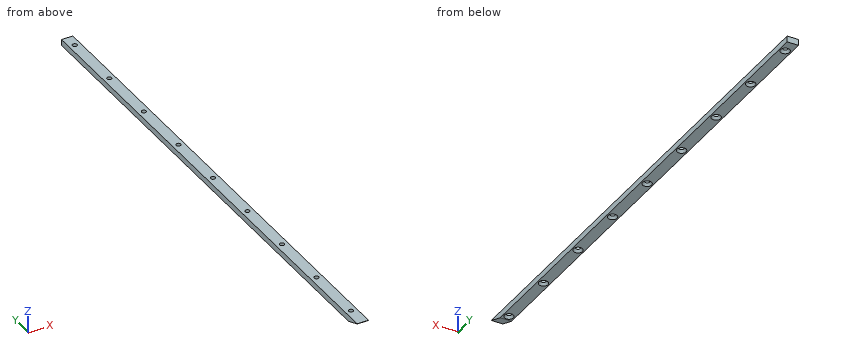
```python
from build123d import *

# Parameters (mm, degrees)
SKETCH1_W           = 15
SKETCH1_H           = 685
BOSS_EXTRUDE1_DEPTH = 4
SKETCH2_R           = 3
CUT_EXTRUDE1_DEPTH  = 8
CHAMFER1_SIZE       = 20
CHAMFER1_SIZE2      = 7.677280701
LPATTERN1_COUNT     = 9
LPATTERN1_PITCH     = 80
CHAMFER2_SIZE       = 3


with BuildPart() as part:
    # Sketch1 → Boss-Extrude1 (new, symmetric)
    with BuildSketch(Plane.XY):
        Rectangle(SKETCH1_W, SKETCH1_H)
    extrude(amount=BOSS_EXTRUDE1_DEPTH, both=True)

    # Sketch2 → Cut-Extrude1 (cut)
    with BuildSketch(Plane.XY.offset(4)):
        with Locations((0, 324.86225561)):
            Circle(SKETCH2_R)
    cut_extrude1 = extrude(amount=-CUT_EXTRUDE1_DEPTH, mode=Mode.SUBTRACT)

    # Chamfer1
    chamfer1_edges = [part.edges().sort_by_distance(p)[0] for p in [
        (0, -342.5, -4),
    ]]
    chamfer1_side = [part.faces().sort_by_distance(p)[0] for p in [
        (0, -0.896409661, -4),
    ]]
    chamfer(chamfer1_edges, length=CHAMFER1_SIZE, length2=CHAMFER1_SIZE2, reference=chamfer1_side[0])

    # LPattern1: Cut-Extrude1 ×9
    with Locations(*[(0, -i * LPATTERN1_PITCH, 0) for i in range(1, LPATTERN1_COUNT)]):
        add(cut_extrude1, mode=Mode.SUBTRACT)

    # Chamfer2
    chamfer2_edges = [part.edges().sort_by_distance(p)[0] for p in [
        (-3, 324.86225561, -4),
        (-3, 244.86225561, -4),
        (-3, 164.86225561, -4),
        (-3, 84.86225561, -4),
        (-3, 4.86225561, -4),
        (-3, -75.13774439, -4),
        (-3, -155.13774439, -4),
        (-3, -235.13774439, -4),
        (-3, -315.13774439, -4),
    ]]
    chamfer(chamfer2_edges, length=CHAMFER2_SIZE)


solid = part.part
```
Here's how the part is built. I have some questions about the finished solid (model axes, mm). Coordinates: 2 decimals unless noted, no trailing zeros.
1) I need wall thicknesses on line 1 (X direction, y = -75.5, z = 3.75). Which ranges of the line are inside material? Lowest first, please.
2) Will this pin go through, and if not, where does the flat tip stop? pin 1 (5.5 mm diameter, centred on x = 0, y = -235.14, fed in from -Z).
3) Imagine slicing it at A-A on z = 1.25. State how many separate pieces and enclosed holes the cut face has, and give its area (3 significant figures).
Response values:
1. line 1: x = -7.5 to -2.98, 2.98 to 7.5
2. pin 1: passes through
3. separate pieces: 1
3. enclosed holes: 9
3. area: 9,930 mm2
